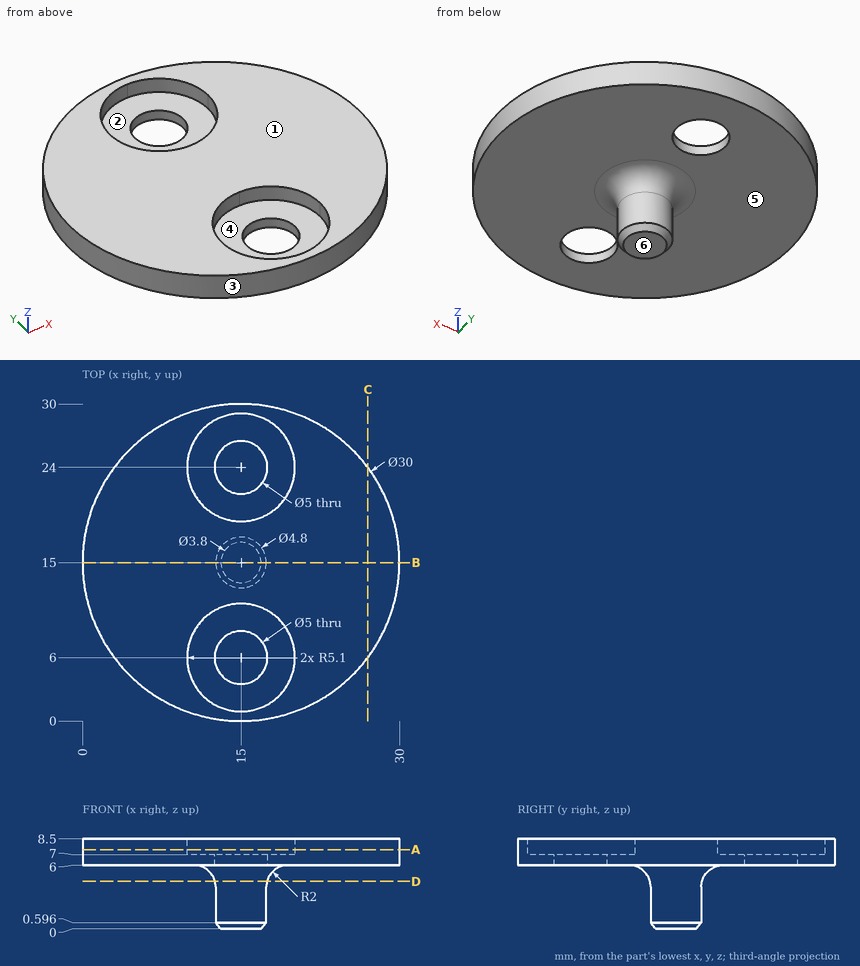
Verification items for this drawing (mm, ordinates from the low corner). A direction names the side the tool comes from. Coordinates: 2 decimals unless noted, no trailing zeros. Order: outer loops, then holes, each group sorted by start corner. A loop starts at its lowest first (then second) coordinate and runs counter-clockwise, first axis right, second up. Notation, with made-up numbers: M 13.5,-12.5 L 69.5,-12.5 A12 cw 69.5,0.5 Z; hole C 26,-31.75 d4. An arc over 180 degrees is marked long. Answer as a JSON object with one key per item and string values.
Q1. Tool access check on the marked faces 4, 5 and 6. Record the directions out of +Z, -Z, +X, -X, +Y, -Y that give a thin tool (end or side, any length) a straight path to the whole face; none if there is none.
Results are:
{"face 4": "+Z", "face 5": "-Z", "face 6": "-Z, +X, -X, +Y, -Y"}
Q2. Depth check by flat-ended pin: pin 1 Ø11 at (x, y) = (15.5, 22.5) entering from +Z; pin 2 Ø4 at (y, z) = (9, 1.5) entering from +X (3 decimals); pin 3 Ø4 at (x, z) = (25, 6.5) entering from -Y; pin 4 Ø1.5 at (x, z) = (12.5, 5.5) entering from +Y. Enter the tip coordinate at first touch or a pass-through.
Results are:
{"pin 1": "stops at z = 8.5", "pin 2": "passes through", "pin 3": "stops at y = 2.31", "pin 4": "stops at y = 29.87"}
Q3. Cross-section at B-B on y = 15. Record the cut outline in (x, z).
Results are:
{"outline": "M 0,6 L 10.6,6 A2 cw 12.6,4 L 12.6,0.6 L 13.1,0 L 16.9,0 L 17.4,0.6 L 17.4,4 A2 cw 19.4,6 L 30,6 L 30,8.5 L 0,8.5 Z"}
Q4. Scan lines: line 1 (Y direction, x = 15, z = 6.3); line 2 (Y direction, x = 14.5, z = 6.75); line 3 (Z direction, x = 26.5, y = 5.5). Record each from-to range of solid material in increasing order.
Results are:
{"line 1": "y = 0 to 3.5, 8.5 to 21.5, 26.5 to 30", "line 2": "y = 0.01 to 3.55, 8.45 to 21.55, 26.45 to 29.99", "line 3": "z = 6 to 8.5"}
Q5. Cross-section at C-C on x = 27. Record the cut outline in (y, z), and give its area (3 significant figures).
Results are:
{"outline": "M 6,6 L 24,6 L 24,8.5 L 6,8.5 Z", "area": "45.0 mm²"}
Q6. Cross-section at A-A on z = 7.5. Record the cut outline in (x, y), and give its area (3 significant figures).
Results are:
{"outline": "C 15,15 d30; hole C 15,6 d10.2; hole C 15,24 d10.2", "area": "543 mm²"}
Q7. Release check for a two-part mould opening along Y. For the marked faces 1, 2 and 3 record: released by +Y, released by -Y, zero draft, split by the parting line, or undercut.
Results are:
{"face 1": "zero draft", "face 2": "undercut", "face 3": "split by the parting line"}
Q8. Cross-section at D-D on z = 4.5. Record the cut outline in (x, y).
Results are:
{"outline": "C 15,15 d4.93"}
